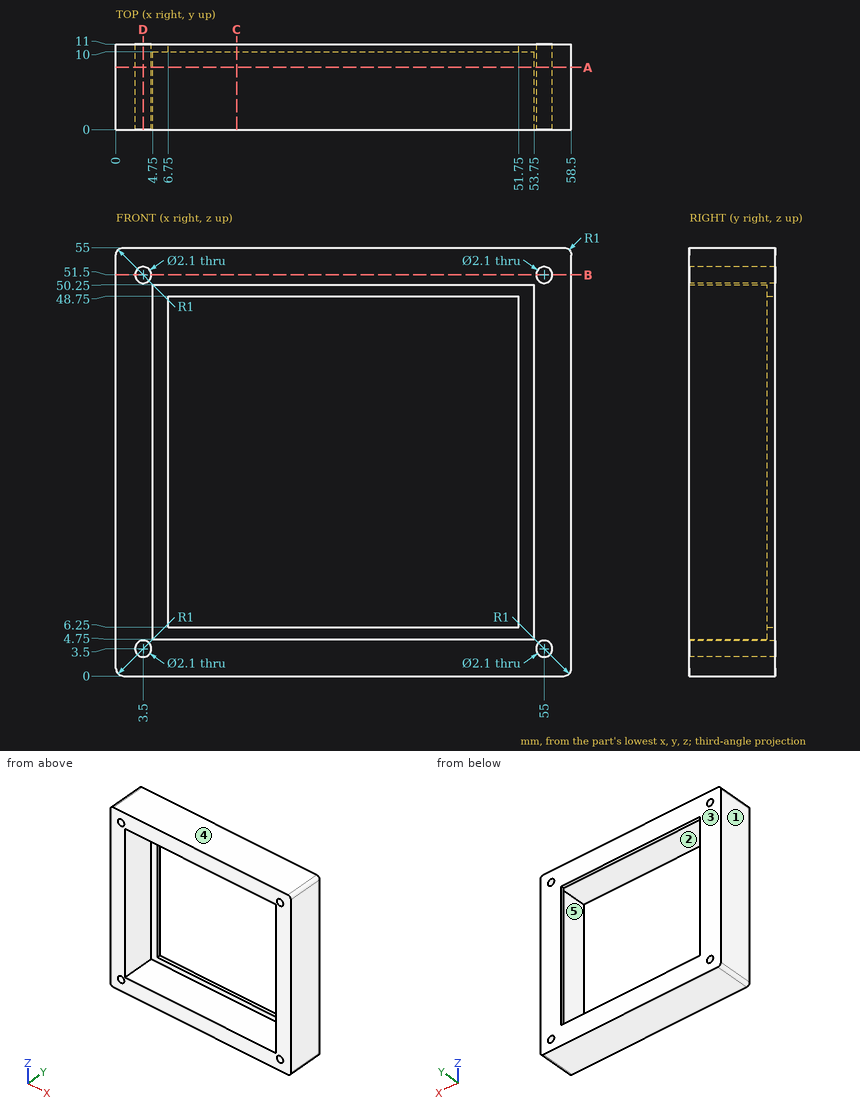
Geometry check sheet. Reference: drawing and pictorial views, mm from the part's lowest x, y, z. A direction names the side the tool comes from. Give positions to 0.01 mm unless a question says otherwise; leave off trailing zeros. Order: outer loops, then holes, each group sorted by start corner. A loop starts at its lowest first (then second) coordinate and runs counter-clockwise, first axis right, second up. Notation, with made-up numbers: (70, 48) - (99, 48) arc R31 ccw to (99, 83) - close; hole circle Ø1 at (-14, 75). An arc over 180 degrees is marked (long way). Use one line per item in the form item = value.
1) Access from +Z, -Z, +X, -X, +Y, -Y to the whole of each face (thin tool, end or side, straight path). Record for the marked faces 1 and 2.
Working result:
face_1 = +Z, -Z, -X, +Y, -Y
face_2 = -Y
2) Sectioned sample at A-A (y = 8). Record the boundary of the cut face in (x, z).
Working result:
outline = (0, 1) arc R1 ccw to (1, 0) - (57.5, 0) arc R1 ccw to (58.5, 1) - (58.5, 54) arc R1 ccw to (57.5, 55) - (1, 55) arc R1 ccw to (0, 54) - close; hole circle Ø2.1 at (3.5, 3.5); hole circle Ø2.1 at (3.5, 51.5); hole (4.75, 4.75) - (53.75, 4.75) - (53.75, 50.25) - (4.75, 50.25) - close; hole circle Ø2.1 at (55, 3.5); hole circle Ø2.1 at (55, 51.5)
3) Sectioned sample at D-D (x = 3.5). Record the boundary of the cut face in (y, z), and give its area (3 significant figures).
Working result:
outline = (0, 0) - (11, 0) - (11, 2.45) - (0, 2.45) - close; (0, 4.55) - (11, 4.55) - (11, 50.45) - (0, 50.45) - close; (0, 52.55) - (11, 52.55) - (11, 55) - (0, 55) - close
area = 559 mm^2
4) Sectioned sample at C-C (x = 15.5). Record the boundary of the cut face in (y, z), and give its area (4 significant figures).
Working result:
outline = (0, 0) - (11, 0) - (11, 6.25) - (10, 6.25) - (10, 4.75) - (0, 4.75) - close; (0, 50.25) - (10, 50.25) - (10, 48.75) - (11, 48.75) - (11, 55) - (0, 55) - close
area = 107.5 mm^2
5) Depth check by flat-ended pin: pin 1 Ø10 at (x, z) = (40.5, 44.5) entering from -Y; pin 2 Ø1.9 at (x, z) = (3.5, 3.5) entering from +Y. Enter the tip coordinate at first touch or a pass-through.
Working result:
pin_1 = 10
pin_2 = through
6) Material ranges on probe 1 along X at (y, z) = (2.5, 51.5); probe 2 along Z at (x, y) = (55, 6.25); probe 3 along X at (y, z) = (7, 28), recorded low to high. Write a range as from..to.
Working result:
probe_1 = 0..2.45, 4.55..53.95, 56.05..58.5
probe_2 = 0..2.45, 4.55..50.45, 52.55..55
probe_3 = 0..4.75, 53.75..58.5
7) Draft check along Z on the marked faces 3, 4 and 5. Enter one of: released by +Z, released by -Z, zero draft, split by the parting line, or undercut.
Working result:
face_3 = zero draft
face_4 = released by +Z
face_5 = undercut
8) Sectioned sample at B-B (z = 51.5). Record the boundary of the cut face in (x, y), and give its area (3 significant figures).
Working result:
outline = (0, 0) - (2.45, 0) - (2.45, 11) - (0, 11) - close; (4.55, 0) - (53.95, 0) - (53.95, 11) - (4.55, 11) - close; (56.05, 0) - (58.5, 0) - (58.5, 11) - (56.05, 11) - close
area = 597 mm^2
